from build123d import *

# Parameters (mm, degrees)
SKETCH_1_W           = 200
SKETCH_1_H           = 213
EXTRUDE_1_DEPTH      = 4
EXTRUDE_2_DEPTH      = 54
CUT_EXTRUDE_2_DEPTH  = 298.880848663
CUT_EXTRUDE_3_DEPTH  = 42
SKETCH_7_R           = 1.8
SKETCH_7_R_2         = 11.5
CUT_EXTRUDE_4_DEPTH  = 282.53330176
MIRROR_START         = 176
MIRROR_1_OUTLINE_R   = 1.8
MIRROR_1_OUTLINE_R_2 = 11.5
MIRROR_1_DEPTH       = 3.5
SKETCH_8_W           = 27
SKETCH_8_H           = 28
CUT_EXTRUDE_5_DEPTH  = 6
SKETCH_9_W           = 27
SKETCH_9_H           = 20
CUT_EXTRUDE_6_DEPTH  = 21
CUT_EXTRUDE_START    = -54
CUT_EXTRUDE_7_DEPTH  = 54
SKETCH_14_W          = 21
SKETCH_14_H          = 20
CUT_EXTRUDE_8_DEPTH  = 296.18299409
SKETCH_15_W          = 6
SKETCH_15_H          = 28
CUT_EXTRUDE_9_DEPTH  = 296.18299409
SKETCH_12_R          = 2.6
CUT_EXTRUDE_10_DEPTH = 8
SKETCH_16_R          = 2.4
CUT_EXTRUDE_11_DEPTH = 3
SKETCH_17_R          = 1.75
CUT_EXTRUDE_12_DEPTH = 20


# Read off the part's stored shape, not the designer's step: 镜向1
with BuildPart() as part:
    # 草图1 → 凸台-拉伸1 (new body)
    with BuildSketch(Plane(origin=(0, 0, 0), x_dir=(1, 0, 0), z_dir=(0, 1, 0))):
        with Locations((100, 106.5)):
            Rectangle(SKETCH_1_W, SKETCH_1_H)
    extrude(amount=EXTRUDE_1_DEPTH)

    # 草图1<4> → 凸台-拉伸2 (add)
    with BuildSketch(Plane(origin=(0, 0, 0), x_dir=(1, 0, 0), z_dir=(0, 1, 0))):
        with BuildLine():
            Line((0, 213), (0, 0))
            ThreePointArc((0, 0), (21.966991411, 53.033008589), (75, 75))
            Line((75, 75), (75, 213))
            Line((75, 213), (0, 213))
        make_face()
        with BuildLine():
            Line((125, 213), (125, 75))
            ThreePointArc((125, 75), (178.033008589, 53.033008589), (200, 0))
            Line((200, 0), (200, 213))
            Line((200, 213), (125, 213))
        make_face()
    extrude(amount=-EXTRUDE_2_DEPTH)

    # 草图3 → 切除-拉伸2 (cut, through all)
    with BuildSketch(Plane.XZ.offset(54)):
        Polygon((20.5, -186), (20.5, -165), (20.5, -144), (20.5, -115), (0, -115), (0, -213), (20.5, -213), align=None)
        Polygon((179.5, -115), (200, -115), (200, -213), (179.5, -213), (179.5, -165), align=None)
    extrude(amount=-CUT_EXTRUDE_2_DEPTH, mode=Mode.SUBTRACT)

    # 草图5 → 切除-拉伸3 (cut)
    with BuildSketch(Plane.XZ.offset(54)):
        Polygon((176, -164), (176, -144), (125, -144), (125, -186), (176, -186), align=None)
        Polygon((24, -164), (24, -144), (75, -144), (75, -186), (24, -186), align=None)
    extrude(amount=-CUT_EXTRUDE_3_DEPTH, mode=Mode.SUBTRACT)

    # 草图7 → 切除-拉伸4 (cut, through all)
    with BuildSketch(Plane(origin=(24, 0, 0), x_dir=(0, 0, -1), z_dir=(1, 0, 0))):
        with Locations((180.5, -17.5)):
            Circle(SKETCH_7_R)
        with Locations((149.5, -17.5)):
            Circle(SKETCH_7_R)
        with Locations((165, -33)):
            Circle(SKETCH_7_R_2)
        with Locations((180.5, -48.5)):
            Circle(SKETCH_7_R)
        with Locations((149.5, -48.5)):
            Circle(SKETCH_7_R)
    extrude(amount=-CUT_EXTRUDE_4_DEPTH, mode=Mode.SUBTRACT)

    # 镜向1 outline → 镜向1 (cut)
    with BuildSketch(Plane.YZ.offset(MIRROR_START)):
        with Locations((-17.5, -180.5)):
            Circle(MIRROR_1_OUTLINE_R)
        with Locations((-17.5, -149.5)):
            Circle(MIRROR_1_OUTLINE_R)
        with Locations((-33, -165)):
            Circle(MIRROR_1_OUTLINE_R_2)
        with Locations((-48.5, -180.5)):
            Circle(MIRROR_1_OUTLINE_R)
        with Locations((-48.5, -149.5)):
            Circle(MIRROR_1_OUTLINE_R)
    extrude(amount=MIRROR_1_DEPTH, mode=Mode.SUBTRACT)

    # 草图8 → 切除-拉伸5 (cut)
    with BuildSketch(Plane(origin=(75, 0, 0), x_dir=(0, 0, -1), z_dir=(1, 0, 0))):
        with Locations((199.5, -33)):
            Rectangle(SKETCH_8_W, SKETCH_8_H)
    extrude(amount=-CUT_EXTRUDE_5_DEPTH, mode=Mode.SUBTRACT)

    # 草图9 → 切除-拉伸6 (cut)
    with BuildSketch(Plane.ZY.offset(-125)):
        with Locations((-199.5, -33)):
            Rectangle(SKETCH_9_W, SKETCH_9_H)
    extrude(amount=-CUT_EXTRUDE_6_DEPTH, mode=Mode.SUBTRACT)

    # 草图11 → 切除-拉伸7 (cut)
    with BuildSketch(Plane.XZ.offset(54).offset(CUT_EXTRUDE_START)):
        with BuildLine():
            Line((29.658534166, -69.684244774), (10.975621098, -39.0625))
            ThreePointArc((10.975621098, -39.0625), (38.289562111, -65.401404801), (75, -75))
            Line((75, -75), (75, -144))
            ThreePointArc((75, -144), (37.483837038, -124.777752739), (31.171635941, -83.099060455))
            ThreePointArc((31.171635941, -83.099060455), (31.899182276, -76.224256342), (29.658534166, -69.684244774))
        make_face()
        with BuildLine():
            Line((125, -144), (125, -75))
            ThreePointArc((125, -75), (161.710437889, -65.401404801), (189.024378902, -39.0625))
            Line((189.024378902, -39.0625), (170.341465834, -69.684244774))
            ThreePointArc((170.341465834, -69.684244774), (168.100817724, -76.224256342), (168.828364059, -83.099060455))
            ThreePointArc((168.828364059, -83.099060455), (162.516162962, -124.777752739), (125, -144))
        make_face()
    extrude(amount=CUT_EXTRUDE_7_DEPTH, mode=Mode.SUBTRACT)

    # 草图14 → 切除-拉伸8 (cut, through all)
    with BuildSketch(Plane.XZ.offset(12)):
        with Locations((64.5, -165)):
            Rectangle(SKETCH_14_W, SKETCH_14_H)
    extrude(amount=-CUT_EXTRUDE_8_DEPTH, mode=Mode.SUBTRACT)

    # 草图15 → 切除-拉伸9 (cut, through all)
    with BuildSketch(Plane.XZ.offset(12)):
        with Locations((128, -165)):
            Rectangle(SKETCH_15_W, SKETCH_15_H)
    extrude(amount=-CUT_EXTRUDE_9_DEPTH, mode=Mode.SUBTRACT)

    # 草图12 → 切除-拉伸10 (cut)
    with BuildSketch(Plane.XZ.offset(54)):
        with Locations(Location((16, -60.517578107, 0), (0, 0, 270))):
            Circle(SKETCH_12_R)
        with Locations(Location((16, -95.517578107, 0), (0, 0, 270))):
            Circle(SKETCH_12_R)
        with Locations(Location((184, -60.517578107, 0), (0, 0, 270))):
            Circle(SKETCH_12_R)
        with Locations(Location((184, -95.517578107, 0), (0, 0, 270))):
            Circle(SKETCH_12_R)
    extrude(amount=-CUT_EXTRUDE_10_DEPTH, mode=Mode.SUBTRACT)

    # 草图16 → 切除-拉伸11 (cut)
    with BuildSketch(Plane.XZ.offset(46)):
        with Locations(Location((184, -95.517578107, 0), (0, 0, 270))):
            Circle(SKETCH_16_R)
        with Locations(Location((184, -60.517578107, 0), (0, 0, 270))):
            Circle(SKETCH_16_R)
        with Locations(Location((16, -60.517578107, 0), (0, 0, 270))):
            Circle(SKETCH_16_R)
        with Locations(Location((16, -95.517578107, 0), (0, 0, 270))):
            Circle(SKETCH_16_R)
    extrude(amount=-CUT_EXTRUDE_11_DEPTH, mode=Mode.SUBTRACT)

    # 草图17 → 切除-拉伸12 (cut)
    with BuildSketch(Plane.XZ.offset(54)):
        with Locations(Location((16, -60.517578107, 0), (0, 0, 270))):
            Circle(SKETCH_17_R)
        with Locations(Location((16, -95.517578107, 0), (0, 0, 270))):
            Circle(SKETCH_17_R)
        with Locations(Location((184, -95.517578107, 0), (0, 0, 270))):
            Circle(SKETCH_17_R)
        with Locations(Location((184, -60.517578107, 0), (0, 0, 270))):
            Circle(SKETCH_17_R)
    extrude(amount=-CUT_EXTRUDE_12_DEPTH, mode=Mode.SUBTRACT)


solid = part.part
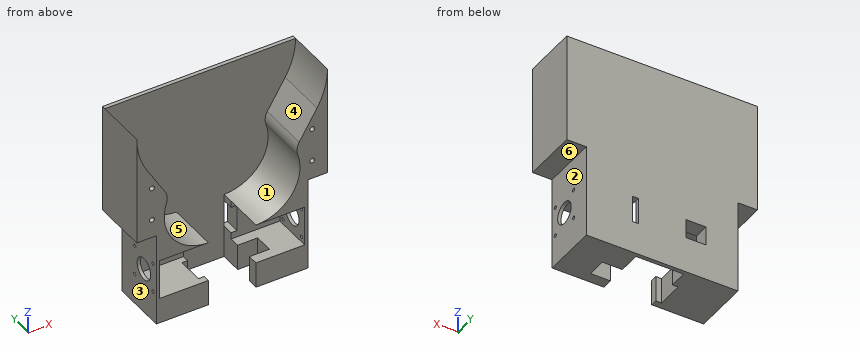
The model under review builds one solid part; all positions refer to its coordinate system, in mm. Face numbers are marked on the shaded views. A direction names the side the tool comes from. Round coordinates to 2 decimals unless told otherwise and drop trailing zeros. Loops run counter-clockwise (first coordinate to the right, second up) from the corner with the lowest first, then second, coordinate; pieces in that order, holes last. Notation, with made-up numbers: (15, 32.25) -> (41, 32.25) arc R11 ccw to (41, 44.25) -> close; hole circle Ø5 at (11, 87). An arc over 180 degrees is marked (long way). Answer as CSV lines item,"result".
1) Draft analysis for pull direction X (two halves, no side actions). For the marked faces 1, 2 and 3, state which applies: pulls with the +X half, pulls with the -X half, needs draft (parallel to the pull), parting line crosses it, or undercut.
Geometry results:
face 1,"undercut"
face 2,"pulls with the +X half"
face 3,"pulls with the -X half"
2) Add section D-D on x = 163. Write out the cut boundary in (y, z), plus the area to 3 significant figures.
Geometry results:
outline,"(-54, -213) -> (4, -213) -> (4, 0) -> (0, 0) -> (0, -124.09) -> (-54, -124.09) -> (-54, -144) -> (-12, -144) -> (-12, -186) -> (-54, -186) -> close"
area,"3,890 mm²"
3) For P1, Ø6.5, axis at x = 126.5, y = -2, coming from the +Z side; P2, Ø4, axis at x = 16, z = -60.5, coming from the -Y side; P3, Ø10, axis at y = -25.5, z = -189, coming from the -X side; P4, Ø8, axis at x = 148, y = -38, coming from the +Z side, all flat-tipped, find the tip position at first contact; note any pin that passes through.
Geometry results:
P1,"stops at z = 0"
P2,"stops at y = -43"
P3,"stops at x = 20.5"
P4,"stops at z = -135.29"
4) Add section C-C on y = -26. State how many separate pieces and enclosed holes the cut face has, plus the area to 3 significant figures.
Geometry results:
separate pieces,"4"
enclosed holes,"0"
area,"8,000 mm²"
5) Add section A-A on z = -165. Write out the cut boundary in (x, y), plus the area to 4 significant figures.
Geometry results:
outline,"(20.5, -54) -> (24, -54) -> (24, -44.5) -> (20.5, -44.5) -> close; (20.5, -21.5) -> (24, -21.5) -> (24, -12) -> (54, -12) -> (54, 4) -> (20.5, 4) -> close; (75, 0) -> (125, 0) -> (125, 4) -> (75, 4) -> close; (131, -12) -> (176, -12) -> (176, -21.5) -> (179.5, -21.5) -> (179.5, 4) -> (131, 4) -> close; (176, -54) -> (179.5, -54) -> (179.5, -44.5) -> (176, -44.5) -> close"
area,"1,645 mm²"
6) To check wall thickness, follow line 1 along Y through (x, z) = (177.05, -180.5); line 2 along Z through (x, y) = (177.4, -17.5); line 3 along Y through (x, z) = (23, -180). State the ranges of each line that lie inside material, in increasing order. Write a range as from..to.
Geometry results:
line 1,"y = -54..-50.3, -46.7..-19.3, -15.7..4"
line 2,"z = -213..-182.3, -178.7..-151.3, -147.7..-58.12"
line 3,"y = -54..-50.23, -46.77..-19.23, -15.77..4"
7) Tool access review of the marked faces 4, 5 and 6: name each direction out of +Z, -Z, +X, -X, +Y, -Y from which nothing blocks a thin tool from reaching the whole face with its end or side.
Geometry results:
face 4,"+Z, -Y"
face 5,"-Y"
face 6,"-Z, +X, +Y, -Y"
8) Add section B-B on x = 61.5. Write out the cut boundary in (y, z).
Geometry results:
outline,"(-54, -213) -> (4, -213) -> (4, -175) -> (-12, -175) -> (-12, -186) -> (-54, -186) -> close; (-54, -144) -> (-12, -144) -> (-12, -155) -> (4, -155) -> (4, 0) -> (0, 0) -> (0, -141.98) -> (-54, -141.98) -> close"
